Verification items for the finished model (mm, model axes). A direction names the side the tool comes from. Give positions to 0.01 mm unless a question says otherwise; leave off trailing zeros. Write each loop counter-clockwise with the first axis right and the second up, starting at its lowest first coordinate (ties: lowest second). Pieces come first, ordered by that corner, then holes. Notation, with made-up numbers: M 19,85.5 L 44,85.5 A18 ccw 44,107.5 Z; hole C -3.5,23.5 d5. An arc over 180 degrees is marked long. Answer as a JSON object with one key per item and string values.
```python
from build123d import *

# Parameters (mm, degrees)
CORTE_EXTRUS_O1_DEPTH = 4
FILETE1_R             = 0.25
FILETE2_R             = 0.25
CHANFRO1_SIZE         = 0.3


with BuildPart() as part:
    # Esboço1 → Revolução1 (revolve)
    with BuildSketch(Plane.XY):
        Polygon((-7.322649731, 3), (-7.122649731, 3), (-6.833974596, 3.5), (-6.433974596, 3.5), (-6.145299462, 3), (-2.5, 3), (-2.5, 4), (1.5, 4), (1.5, 2.25), (7.5, 2.25), (7.5, 1.75), (-3.200961894, 1.75), (-4.5, 2.5), (-8.5, 2.5), (-8.5, 3), (-8.3, 3), (-8.011324865, 3.5), (-7.611324865, 3.5), align=None)
    revolve(axis=Axis((-29.721905334, 0, 0), (1, 0, 0)))

    # Esboço2 → Corte-extrusão1 (cut)
    with BuildSketch(Plane(origin=(1.5, 0, 0), x_dir=(0, 0, -1), z_dir=(1, 0, 0))):
        with BuildLine():
            Line((-2, 3.464101615), (2, 3.464101615))
            ThreePointArc((2, 3.464101615), (0, 4), (-2, 3.464101615))
        make_face()
        with BuildLine():
            Line((-4, 0), (-2, 3.464101615))
            ThreePointArc((-2, 3.464101615), (-3.464101615, 2), (-4, 0))
        make_face()
        with BuildLine():
            ThreePointArc((-4, 0), (-3.464101615, -2), (-2, -3.464101615))
            Line((-2, -3.464101615), (-4, 0))
        make_face()
        with BuildLine():
            ThreePointArc((-2, -3.464101615), (0, -4), (2, -3.464101615))
            Line((2, -3.464101615), (-2, -3.464101615))
        make_face()
        with BuildLine():
            ThreePointArc((2, -3.464101615), (3.464101615, -2), (4, 0))
            Line((4, 0), (2, -3.464101615))
        make_face()
        with BuildLine():
            Line((2, 3.464101615), (4, 0))
            ThreePointArc((4, 0), (3.464101615, 2), (2, 3.464101615))
        make_face()
    extrude(amount=-CORTE_EXTRUS_O1_DEPTH, mode=Mode.SUBTRACT)

    # Filete1
    filete1_edges = [part.edges().sort_by_distance(p)[0] for p in [
        (-8.011324865, -3.5, 0),
        (-7.611324865, -3.5, 0),
    ]]
    fillet(filete1_edges, radius=FILETE1_R)

    # Filete2
    filete2_edges = [part.edges().sort_by_distance(p)[0] for p in [
        (-6.833974596, -3.5, 0),
        (-6.433974596, -3.5, 0),
    ]]
    fillet(filete2_edges, radius=FILETE2_R)

    # Chanfro1
    chanfro1_edges = [part.edges().sort_by_distance(p)[0] for p in [
        (7.5, -1.75, 0),
    ]]
    chamfer(chanfro1_edges, length=CHANFRO1_SIZE)


solid = part.part
```
1) Access from +Z, -Z, +X, -X, +Y, -Y to the whole of each face (thin tool, end or side, straight path). Record for faces 1 (the face through (-0.472, -1.708, -3.014)), 2 (the face through (-2.5, -1, -3)), 3 (the face through (4.54, -0.29, 2.23)).
Completed:
{"face 1": "-Z, +X, -Y", "face 2": "none", "face 3": "+X"}
2) Thickness scan on L1, parallel to Z at x = -5.9, y = 0; L2, parallel to X at y = 1, z = -3; L3, parallel to Y at x = 1.25, z = 0.5. Record the ranges inside material, lowest first.
Completed:
{"L1": "z = -3 to -2.5, 2.5 to 3", "L2": "x = -8.21 to -7.42, -7.03 to -6.24, -2.5 to 1.5", "L3": "y = -3.46 to -1.68, 1.68 to 3.46"}
3) Release check for a two-part mould opening along Z. For faces 4 (the face through (-0.472, 1.708, 3.014)), 5 (the face through (1.5, -2, -2)), 6 (the face through (1.927, 1.617, -0.67)) record: pulls with the +Z half, pulls with the -Z half, needs draft (parallel to the pull), parting line crosses it, or undercut.
Completed:
{"face 4": "pulls with the +Z half", "face 5": "needs draft", "face 6": "undercut"}
4) Go/stop test with flat-tipped pins: pin 1 (1.5 mm diameter, centred on x = -4.5, y = 1.5, fed in from +Z); pin 2 (3 mm diameter, centred on x = 2.5, z = -1.5, fed in from -Y); pin 3 (1.5 mm diameter, centred on x = 3, y = -1.5, fed in from +Z). Record where each tip stops, or that it passes through.
Completed:
{"pin 1": "stops at z = 2.9", "pin 2": "stops at y = -3.46", "pin 3": "stops at z = 2.12"}
5) Section check A-A on x = -1.5. Record the boundary of the cut face in (y, z).
Completed:
{"outline": "M -3.46,-2 L 0,-4 L 3.46,-2 L 3.46,2 L 0,4 L -3.46,2 Z; hole C 0,0 d3.5"}
6) Section check B-B on x = 3.25. Record the boundary of the cut face in (y, z).
Completed:
{"outline": "C 0,0 d4.5; hole C 0,0 d3.5"}
